Geometry: final body of the model. Coordinates: model frame, mm. Face numbers are marked on the shaded views. A direction names the side the tool comes from. Round coordinates to 2 decimals unless told otherwise and drop trailing zeros. Write each loop counter-clockwise with the first axis right and the second up, starting at its lowest first coordinate (ties: lowest second). Pieces come first, ordered by that corner, then holes. Notation, with made-up numbers: M 3.5,35.25 L 61.5,35.25 A15 cw 61.5,43.25 Z; hole C 0,-28 d1. An arc over 180 degrees is marked long. Use one line per item in the form item = value. Start each with the question number.
Item 1: Ray query, probe 1 along Z at (x, y) = (-5.85, 0); probe 2 along Y at (x, z) = (0, 10). Return the intervals inside material, ascending.
Item 2: Section query B-B (z = 3.75). Return loops of the section in (x, y), and give its area (3 significant figures).
Item 3: Pin query (flat end, axial travel): pin 1 Ø2.5 at (x, y) = (4.5, -1.5) entering from +Z; pin 2 Ø2 at (x, y) = (-2, 5.5) entering from +Z; pin 3 Ø2 at (x, z) = (-3, 7) entering from +Y. Return the tip coordinate at first contact, or that it passes through.
Item 4: Section query C-C (x = -4.25). Return loops of the section in (y, z), and give its area (3 significant figures).
Item 5: Section query D-D (z = 8). Return loops of the section in (x, y), and give its area (3 significant figures).
Item 6: Pull-direction query (X, two-part tool) for the marked faces 1, 2 and 3; classes: pulls with the +X half, pulls with the -X half, needs draft (parallel to the pull), parting line crosses it, or undercut.
Item 7: Section query A-A (y = 0). Return loops of the section in (x, z), and give its area (4 significant figures).
Item 8: Reachability of the marked faces 4 and 5 from +Z, -Z, +X, -X, +Y, -Y: full face, straight path, thin tool, end or side. Return the list, or none.
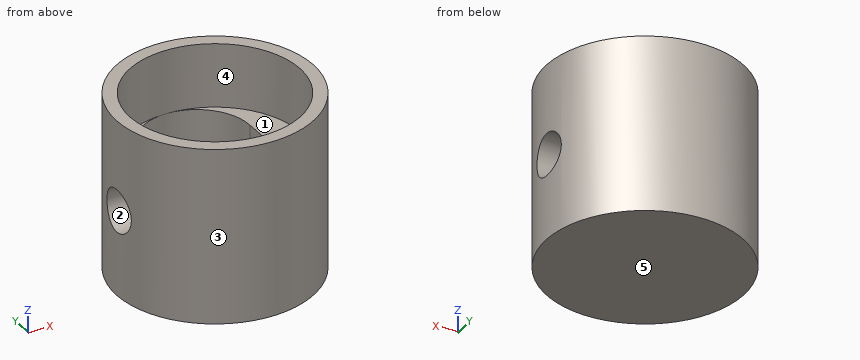
from build123d import *

# Parameters (mm, degrees)
ESQUISSE1_R             = 9.25
BASE_EXTRUSION_DEPTH    = 16.5
ESQUISSE2_R             = 2
ENL_V_MAT_EXTRU_1_DEPTH = 27.458694223
ESQUISSE3_R             = 8
ENL_V_MAT_EXTRU_2_DEPTH = 6
ENL_V_MAT_EXTRU_3_DEPTH = 10


with BuildPart() as part:
    # Esquisse1 → Base-Extrusion (new body)
    with BuildSketch(Plane.XY):
        Circle(ESQUISSE1_R)
    extrude(amount=BASE_EXTRUSION_DEPTH)

    # Esquisse2 → Enlèv. mat.-Extru.1 (cut, through all)
    with BuildSketch(Plane(origin=(9.25, 0, 0), x_dir=(0, 0, -1), z_dir=(1, 0, 0))):
        with Locations((-8, 0)):
            Circle(ESQUISSE2_R)
    extrude(amount=-ENL_V_MAT_EXTRU_1_DEPTH, mode=Mode.SUBTRACT)

    # Esquisse3 → Enlèv. mat.-Extru.2 (cut)
    with BuildSketch(Plane.XY.offset(16.5)):
        Circle(ESQUISSE3_R)
    extrude(amount=-ENL_V_MAT_EXTRU_2_DEPTH, mode=Mode.SUBTRACT)

    # Esquisse4 → Enlèv. mat.-Extru.3 (cut)
    with BuildSketch(Plane.XY.offset(10.5)):
        with BuildLine():
            Line((5, 3), (5, -3))
            ThreePointArc((5, -3), (0, -8), (-5, -3))
            Line((-5, -3), (-5, 3))
            ThreePointArc((-5, 3), (0, 8), (5, 3))
        make_face()
    extrude(amount=-ENL_V_MAT_EXTRU_3_DEPTH, mode=Mode.SUBTRACT)


solid = part.part
Working result:
q1.probe_1 = 0 to 6, 10 to 10.5
q1.probe_2 = -9.25 to -8, 8 to 9.25
q2.outline = C 0,0 d18.5; hole M -5,-3 A5 ccw 5,-3 L 5,3 A5 ccw -5,3 Z
q2.area = 130 mm²
q3.pin_1 = 10.5
q3.pin_2 = 0.5
q3.pin_3 = 9.03
q4.outline = M -8.22,0 L 8.22,0 L 8.22,16.5 L 6.78,16.5 L 6.78,10.5 L 5.63,10.5 L 5.63,0.5 L -5.63,0.5 L -5.63,10.5 L -6.78,10.5 L -6.78,16.5 L -8.22,16.5 Z
q4.area = 77.1 mm²
q5.outline = M -9.03,-2 A9.25 ccw 9.03,-2 L 5,-2 L 5,-3 A5 cw -5,-3 L -5,-2 Z; M -9.03,2 L -5,2 L -5,3 A5 cw 5,3 L 5,2 L 9.03,2 A9.25 ccw Z
q5.area = 96.8 mm²
q6.face_1 = undercut
q6.face_2 = needs draft
q6.face_3 = parting line crosses it
q7.outline = M -9.25,0 L 9.25,0 L 9.25,6 L 5,6 L 5,0.5 L -5,0.5 L -5,6 L -9.25,6 Z; M -9.25,10 L -5,10 L -5,10.5 L -8,10.5 L -8,16.5 L -9.25,16.5 Z; M 5,10 L 9.25,10 L 9.25,16.5 L 8,16.5 L 8,10.5 L 5,10.5 Z
q7.area = 75.25 mm²
q8.face_4 = +Z
q8.face_5 = -Z, +X, -X, +Y, -Y
